The listing builds one solid part. Answer for the finished solid, in the listing's coordinates (mm). A direction names the side the tool comes from. Round coordinates to 2 decimals unless told otherwise and drop trailing zeros. Loops run counter-clockwise (first coordinate to the right, second up) from the corner with the lowest first, then second, coordinate; pieces in that order, holes last. Notation, with made-up numbers: (12.25, 68) -> (27.25, 68) arc R28 ccw to (27.25, 89) -> close; hole circle Ø6 at (20, 15.25). An arc over 180 degrees is marked (long way). Use a Markdown table: item, result. Add a question column.
Q1. For a pull along Z with two mould halves and no side action, classify faces 3 (the flat face through (0, 0.503, 4)), 4 (the cylindrical face through (0.034, 0.814, 1.236)), 5 (the flat face through (0.881, 0.592, -1.264)) as released by +Z, released by -Z, zero draft, split by the parting line, or undercut.
Q2. Given pin 1 Ø1.1 at (x, z) = (0, -3) entering from +Y; pin 2 Ø1.1 at (x, z) = (0, 4) entering from -Y, each flat-ended and moving along its own axis, determine where each tip first touches the part or whether it passes through.
Q3. Section B-B on y = 0.8 is taken. Give the vertices of the cut face in (x, z) (3 decimals).
Q4. Section D-D on z = 4 is taken. Give the vertices of the cut face in (x, y), then the cut area to 3 significant figures.
Q5. Which of the six approach directions +Z, -Z, +X, -X, +Y, -Y give full straight-line access (tool end or side, diameter ignored) to faces 1 (the flat face through (1, 0, 0)), 2 (the flat face through (0, 0.501, -3))?
Q6. Section C-C on z = 0 is taken. Give the vertices of the cut face in (x, y).
Q7. Consider line 1 (X direction, y = 0.5, z = 0); line 2 (Y direction, x = 0.3, z = 3.5); line 3 (X direction, y = 0.15, z = -2.75). Determine where each line is inside the solid, lowest interval first.
Q8. Section A-A on z = 2 is taken. Give the vertices of the cut face in (x, y) (3 decimals), then the cut area to 3 significant figures.
from build123d import *

# Parameters (mm, degrees)
SKETCH1_W           = 2.5
SKETCH1_H           = 6.5
BOSS_EXTRUDE1_DEPTH = 1.2
SKETCH2_R           = 0.6
SKETCH2_R_2         = 0.765
SKETCH2_R_3         = 0.4
CUT_EXTRUDE1_DEPTH  = 1.2
CHAMFER1_SIZE       = 3
CHAMFER1_SIZE2      = 1.091910703
CHAMFER2_SIZE       = 3
CHAMFER2_SIZE2      = 1.091910703
SKETCH3_W           = 2.5
SKETCH3_H           = 1.2
CUT_EXTRUDE2_DEPTH  = 1
CHAMFER3_SIZE       = 0.3
CHAMFER3_SIZE2      = 0.519615242
FILLET1_R           = 0.1
SKETCH4_W           = 1
SKETCH4_H           = 0.5
BOSS_EXTRUDE2_DEPTH = 1
SKETCH5_W           = 2
SKETCH5_H           = 0.5
BOSS_EXTRUDE3_DEPTH = 1
SKETCH6_W           = 0.5
SKETCH6_H           = 0.25
BOSS_EXTRUDE4_DEPTH = 0.5
SKETCH8_W           = 1
SKETCH8_H           = 0.25
BOSS_EXTRUDE6_DEPTH = 0.5
SKETCH9_W           = 2.896936236
SKETCH9_H           = 1.571826666
CUT_EXTRUDE3_DEPTH  = 129.011727979


# Read off the part's stored shape, not the designer's step: Mirror2, Mirror4, Mirror6, Mirror7
with BuildPart() as part:
    # Sketch1 → Boss-Extrude1 (new body)
    with BuildSketch(Plane(origin=(0, 0, 0), x_dir=(1, 0, 0), z_dir=(0, 1, 0))):
        Rectangle(SKETCH1_W, SKETCH1_H)
    extrude(amount=BOSS_EXTRUDE1_DEPTH)

    # Sketch2 → Cut-Extrude1 (cut)
    with BuildSketch(Plane(origin=(0, 1.2, 0), x_dir=(1, 0, 0), z_dir=(0, 1, 0))):
        with Locations(Location((0, 0, 0), (0, 0, 270))):
            Circle(SKETCH2_R)
        with Locations(Location((0, -2, 0), (0, 0, 270))):
            Circle(SKETCH2_R_2)
        with Locations(Location((-0.001766606, 1.5, 0), (0, 0, 270))):
            Circle(SKETCH2_R_3)
    extrude(amount=-CUT_EXTRUDE1_DEPTH, mode=Mode.SUBTRACT)

    # Chamfer1
    chamfer1_edges = [part.edges().sort_by_distance(p)[0] for p in [
        (1.25, 0.6, -3.25),
    ]]
    chamfer1_side = [part.faces().sort_by_distance(p)[0] for p in [
        (1.25, 0.6, 0),
    ]]
    chamfer(chamfer1_edges, length=CHAMFER1_SIZE, length2=CHAMFER1_SIZE2, reference=chamfer1_side[0])

    # Chamfer2
    chamfer2_edges = [part.edges().sort_by_distance(p)[0] for p in [
        (-1.25, 0.6, -3.25),
    ]]
    chamfer2_side = [part.faces().sort_by_distance(p)[0] for p in [
        (-1.25, 0.6, 0),
    ]]
    chamfer(chamfer2_edges, length=CHAMFER2_SIZE, length2=CHAMFER2_SIZE2, reference=chamfer2_side[0])

    # Sketch3 → Cut-Extrude2 (cut)
    with BuildSketch(Plane(origin=(0, 0, -3.25), x_dir=(-1, 0, 0), z_dir=(0, 0, -1))):
        with Locations((0, 0.6)):
            Rectangle(SKETCH3_W, SKETCH3_H)
    extrude(amount=-CUT_EXTRUDE2_DEPTH, mode=Mode.SUBTRACT)

    # Chamfer3
    chamfer3_edges = [part.edges().sort_by_distance(p)[0] for p in [
        (0, 0, 1.235),
    ]]
    chamfer3_side = [part.faces().sort_by_distance(p)[0] for p in [
        (0.000100657, 0, 0.709259096),
    ]]
    chamfer(chamfer3_edges, length=CHAMFER3_SIZE, length2=CHAMFER3_SIZE2, reference=chamfer3_side[0])

    # Fillet1
    fillet1_edges = [part.edges().sort_by_distance(p)[0] for p in [
        (0, 0, -0.6),
        (0, 1.2, -0.6),
        (0, 1.2, 1.235),
        (-0.001766606, 0, -1.9),
        (-0.001766606, 1.2, -1.9),
    ]]
    fillet(fillet1_edges, radius=FILLET1_R)

    # Sketch4 → Boss-Extrude2 (add)
    with BuildSketch(Plane(origin=(0, 0, -2.25), x_dir=(-1, 0, 0), z_dir=(0, 0, -1))):
        with Locations((0, 0.250555681)):
            Rectangle(SKETCH4_W, SKETCH4_H)
    extrude(amount=BOSS_EXTRUDE2_DEPTH)

    # Sketch5 → Boss-Extrude3 (add)
    with BuildSketch(Plane.XY.offset(3.25)):
        with Locations((0, 0.252908482)):
            Rectangle(SKETCH5_W, SKETCH5_H)
    extrude(amount=BOSS_EXTRUDE3_DEPTH)

    # Sketch6 → Boss-Extrude4 (add)
    with BuildSketch(Plane(origin=(0, 0, -3.25), x_dir=(-1, 0, 0), z_dir=(0, 0, -1))):
        with Locations((0, 0.250555681)):
            Rectangle(SKETCH6_W, SKETCH6_H)
    extrude(amount=BOSS_EXTRUDE4_DEPTH)

    # Sketch8 → Boss-Extrude6 (add)
    with BuildSketch(Plane.XY.offset(4.25)):
        with Locations((0, 0.252908482)):
            Rectangle(SKETCH8_W, SKETCH8_H)
    extrude(amount=BOSS_EXTRUDE6_DEPTH)

    # Mirror2: part across plane


with BuildPart() as part_1:
    add(part.part)
    add(part.part.mirror(Plane(origin=(0, 0, 4.75), x_dir=(1, 0, 0), z_dir=(0, 0, -1))))

    # Mirror4: part across plane


with BuildPart() as part_2:
    add(part_1.part)
    add(part_1.part.mirror(Plane.XY.offset(13.25)))

    # Mirror6: part across plane


with BuildPart() as part_3:
    add(part_2.part)
    add(part_2.part.mirror(Plane.XY.offset(30.25)))

    # Mirror7: part across plane


with BuildPart() as part_4:
    add(part_3.part)
    add(part_3.part.mirror(Plane.XY.offset(64.25)))

    # Sketch9 → Cut-Extrude3 (cut, through all)
    with BuildSketch(Plane.XY.offset(4.25)):
        with Locations((0.013927578, 0.592041384)):
            Rectangle(SKETCH9_W, SKETCH9_H)
    extrude(amount=CUT_EXTRUDE3_DEPTH, mode=Mode.SUBTRACT)


solid = part_4.part
Checked values:
| question | item | result |
|---|---|---|
| 1 | face 3 | zero draft |
| 1 | face 4 | undercut |
| 1 | face 5 | released by -Z |
| 2 | pin 1 | stops at y = 0.5 |
| 2 | pin 2 | stops at y = 0 |
| 3 | outline | (-1.25, -0.25) -> (-0.522, -2.25) -> (0.522, -2.25) -> (1.25, -0.25) -> (1.25, 3.25) -> (-1.25, 3.25) -> close; hole circle Ø1.53 at (0, 2); hole circle Ø1.2 at (0, 0); hole circle Ø0.8 at (-0.002, -1.5) |
| 4 | outline | (-1, 0) -> (1, 0) -> (1, 0.5) -> (-1, 0.5) -> close |
| 4 | area | 1.00 mm2 |
| 5 | face 1 | +Z, -Z, +X, -X, -Y |
| 5 | face 2 | -Z, +X, -X, +Y |
| 6 | outline | (-1.25, 0) -> (-0.7, 0) arc R0.1 ccw to (-0.6, 0.1) -> (-0.6, 1.1) arc R0.1 ccw to (-0.7, 1.2) -> (-1.25, 1.2) -> close; (0.6, 0.1) arc R0.1 ccw to (0.7, 0) -> (1.25, 0) -> (1.25, 1.2) -> (0.7, 1.2) arc R0.1 ccw to (0.6, 1.1) -> close |
| 7 | line 1 | x = -1.25 to -0.6, 0.6 to 1.25 |
| 7 | line 2 | y = 0 to 0.5 |
| 7 | line 3 | x = -0.5 to 0.5 |
| 8 | outline | (-1.25, 0) -> (-1.065, 0) -> (-0.765, 0.52) -> (-0.765, 1.1) arc R0.1 ccw to (-0.865, 1.2) -> (-1.25, 1.2) -> close; (0.765, 0.52) -> (1.065, 0) -> (1.25, 0) -> (1.25, 1.2) -> (0.865, 1.2) arc R0.1 ccw to (0.765, 1.1) -> close |
| 8 | area | 1.00 mm2 |
